Here's how the part is built. I have some questions about the finished solid (model axes, mm). A direction names the side the tool comes from. Coordinates: 2 decimals unless noted, no trailing zeros. Write each loop counter-clockwise with the first axis right and the second up, starting at its lowest first coordinate (ties: lowest second). Pieces come first, ordered by that corner, then holes.
```python
from build123d import *

# Parameters (mm, degrees)
F1_DEPTH = 136.652


with BuildPart() as f1:
    # F0 (on Front) → F1 (new body)
    with BuildSketch(Plane.XZ):
        with BuildLine():
            ThreePointArc((54.527499783, 20.9989734618), (54.7276679048, 20.7850152309), (54.9257769328, 20.5691490349))
            ThreePointArc((54.9257769328, 20.5691490349), (76.1901987299, 13.7983190429), (93.7294736505, 0))
            ThreePointArc((93.7294736505, 0), (99.5048519531, 7.4078439529), (104.1196596047, 15.589206731))
            ThreePointArc((104.1196596047, 15.589206731), (77.9936820742, 70.717129744), (25.6797344721, 102.1003335947))
            ThreePointArc((25.6797344721, 102.1003335947), (11.7801687474, 95.1325271586), (0, 84.9848240614))
            ThreePointArc((0, 84.9848240614), (8.2911620822, 73.9876177792), (13.9425107784, 61.4279930793))
            ThreePointArc((13.9425107784, 61.4279930793), (18.3589234819, 58.8669445911), (22.3165845225, 55.6419500772))
            ThreePointArc((22.3165845225, 55.6419500772), (45.1535066394, 46.1825872135), (54.6128695031, 23.3456650966))
            ThreePointArc((54.6128695031, 23.3456650966), (54.5915200165, 22.1715431248), (54.527499783, 20.9989734618))
        make_face()
        with BuildLine():
            ThreePointArc((93.7294736505, 0), (76.7382859544, -13.2702968374), (56.2774381887, -20.0640400021))
            ThreePointArc((56.2774381887, -20.0640400021), (56.3045635593, -20.8278500085), (56.3136070377, -21.5920880129))
            ThreePointArc((56.3136070377, -21.5920880129), (47.4391029946, -43.8287739455), (25.6927352215, -53.8448865624))
            ThreePointArc((25.6927352215, -53.8448865624), (19.5331456536, -59.5527538305), (12.1485373896, -63.5512351899))
            ThreePointArc((12.1485373896, -63.5512351899), (6.9976805403, -73.8751515766), (0, -83.0483213067))
            ThreePointArc((0, -83.0483213067), (12.9593131443, -94.1642757812), (28.4396211824, -101.3662410752))
            ThreePointArc((28.4396211824, -101.3662410752), (78.7986877851, -69.8190066246), (104.0530293111, -16.027912337))
            ThreePointArc((104.0530293111, -16.027912337), (99.5048519531, -7.6187369724), (93.7294736505, 0))
        make_face()
        with BuildLine():
            ThreePointArc((104.1196596047, 15.589206731), (99.5048519531, 7.4078439529), (93.7294736505, 0))
            ThreePointArc((93.7294736505, 0), (99.5048519531, -7.6187369724), (104.0530293111, -16.027912337))
            ThreePointArc((104.0530293111, -16.027912337), (104.9729816843, -8.0374124574), (105.2802302558, 0))
            ThreePointArc((105.2802302558, 0), (104.9896866841, 7.816173788), (104.1196596047, 15.589206731))
        make_face()
        with BuildLine():
            ThreePointArc((109.4791079844, -41.5241606534), (108.1075668029, -28.4905405885), (104.0530293111, -16.027912337))
            ThreePointArc((104.0530293111, -16.027912337), (78.7986877851, -69.8190066246), (28.4396211824, -101.3662410752))
            ThreePointArc((28.4396211824, -101.3662410752), (84.0593765341, -91.8939755487), (109.4791079844, -41.5241606534))
        make_face()
        with BuildLine():
            ThreePointArc((25.6797344721, 102.1003335947), (77.9936820742, 70.717129744), (104.1196596047, 15.589206731))
            ThreePointArc((104.1196596047, 15.589206731), (108.6056945653, 28.7097136295), (110.1253773364, 42.4924120307))
            ThreePointArc((110.1253773364, 42.4924120307), (83.3457717598, 94.174543643), (25.6797344721, 102.1003335947))
        make_face()
        with BuildLine():
            ThreePointArc((-56.3136070377, -21.5920880129), (-57.9095553347, -19.6725800372), (-59.3524805988, -17.6355408825))
            ThreePointArc((-59.3524805988, -17.6355408825), (-75.8807124036, -11.0348961584), (-89.8443087935, 0))
            ThreePointArc((-89.8443087935, 0), (-97.5622695247, -10.3588890688), (-102.9329187465, -22.1074901568))
            ThreePointArc((-102.9329187465, -22.1074901568), (-77.3108882291, -71.4629515478), (-30.118879838, -100.8800275576))
            ThreePointArc((-30.118879838, -100.8800275576), (-13.7568828123, -94.1642757812), (0, -83.0483213067))
            ThreePointArc((0, -83.0483213067), (-6.7178829074, -73.9195667822), (-11.6800359007, -63.7293191111))
            ThreePointArc((-11.6800359007, -63.7293191111), (-19.3289034102, -59.6979704443), (-25.6927352215, -53.8448865624))
            ThreePointArc((-25.6927352215, -53.8448865624), (-47.4391029946, -43.8287739455), (-56.3136070377, -21.5920880129))
        make_face()
        with BuildLine():
            ThreePointArc((-30.118879838, -100.8800275576), (-0.874115727, -105.2766014098), (28.4396211824, -101.3662410752))
            ThreePointArc((28.4396211824, -101.3662410752), (12.9593131443, -94.1642757812), (0, -83.0483213067))
            ThreePointArc((0, -83.0483213067), (-13.7568828123, -94.1642757812), (-30.118879838, -100.8800275576))
        make_face()
        with BuildLine():
            ThreePointArc((0, 84.9848240614), (11.7801687474, 95.1325271586), (25.6797344721, 102.1003335947))
            ThreePointArc((25.6797344721, 102.1003335947), (-0.7599031291, 105.2774877642), (-27.1509221895, 101.7189967851))
            ThreePointArc((-27.1509221895, 101.7189967851), (-12.4779975244, 95.1325271586), (0, 84.9848240614))
        make_face()
        with BuildLine():
            ThreePointArc((-102.9329187465, -22.1074901568), (-97.5622695247, -10.3588890688), (-89.8443087935, 0))
            ThreePointArc((-89.8443087935, 0), (-97.5622695247, 10.0482551584), (-103.0701310001, 21.4586807219))
            ThreePointArc((-103.0701310001, 21.4586807219), (-105.2797080994, -0.3315798868), (-102.9329187465, -22.1074901568))
        make_face()
        with BuildLine():
            ThreePointArc((-103.0701310001, 21.4586807219), (-97.5622695247, 10.0482551584), (-89.8443087935, 0))
            ThreePointArc((-89.8443087935, 0), (-75.8216360442, 11.2724103293), (-59.1261791661, 17.977953208))
            ThreePointArc((-59.1261791661, 17.977953208), (-57.0156534005, 20.7846782143), (-54.6128695031, 23.3456650966))
            ThreePointArc((-54.6128695031, 23.3456650966), (-45.1535066394, 46.1825872135), (-22.3165845225, 55.6419500772))
            ThreePointArc((-22.3165845225, 55.6419500772), (-18.1199759802, 59.0304671081), (-13.4179508285, 61.6732933224))
            ThreePointArc((-13.4179508285, 61.6732933224), (-7.9622593488, 74.0504399858), (0, 84.9848240614))
            ThreePointArc((0, 84.9848240614), (-12.4779975244, 95.1325271586), (-27.1509221895, 101.7189967851))
            ThreePointArc((-27.1509221895, 101.7189967851), (-76.4840523057, 72.3471950086), (-103.0701310001, 21.4586807219))
        make_face()
        with BuildLine():
            ThreePointArc((-102.9329187465, -22.1074901568), (-89.8443087935, -83.0483213067), (-30.118879838, -100.8800275576))
            ThreePointArc((-30.118879838, -100.8800275576), (-77.3108882291, -71.4629515478), (-102.9329187465, -22.1074901568))
        make_face()
        with BuildLine():
            ThreePointArc((-103.0701310001, 21.4586807219), (-76.4840523057, 72.3471950086), (-27.1509221895, 101.7189967851))
            ThreePointArc((-27.1509221895, 101.7189967851), (-89.8443087935, 84.9848240614), (-103.0701310001, 21.4586807219))
        make_face()
    extrude(amount=F1_DEPTH)


solid = f1.part
```
1) I need wall thicknesses on probe 1 along X at (y, z) = (-52.5, -45); probe 2 along Z at (x, y) = (-59, -54.5); probe 3 along X at (y, z) = (-68, -63). Which ranges of each line are inside material? Lowest first, please.
Values follow:
probe 1: x = -106 to -46.27, 46.27 to 109.38
probe 2: z = -101.06 to -18.16, 18.16 to 102.7
probe 3: x = -102.2 to -13.48, 13.48 to 105.68
2) On a 3-axis mill with a long thin cutter (end or side, diameter ignored), from which of +Z, -Z, +X, -X, +Y, -Y can I reach the whole of each face in a straight line? I mean faces 1 (the face through (-75.66, -67.37, -11.16)), 2 (the face through (48, -136.652, 49)). Say none if no direction works.
Values follow:
face 1: +Y, -Y
face 2: +Z, -Z, +X, -X, -Y
3) We'd pull the mould along Z, two halves only. Please class faces 3 (the face through (48, 0, 49)), 4 (the face through (-105.28, -67.37, -0.02)): pulls with the +Z half, pulls with the -Z half, needs draft (parallel to the pull), parting line crosses it, or undercut.
Values follow:
face 3: needs draft
face 4: undercut
4) Imagine slicing it at C-C on y = -43.5. Please give me the cut outline in (x, z), then the cut area to 3 significant figures.
Values follow:
outline: (-103.07, 21.46) arc R105.28 ccw to (-102.93, -22.11) arc R61.17 ccw to (-30.12, -100.88) arc R105.28 ccw to (28.44, -101.37) arc R62.61 ccw to (104.05, -16.03) arc R105.28 ccw to (104.12, 15.59) arc R63.26 ccw to (25.68, 102.1) arc R105.28 ccw to (-27.15, 101.72) arc R61.84 ccw to start; hole (-89.84, 0) arc R61.84 ccw to (-59.35, -17.64) arc R32.3 ccw to (-56.31, -21.59) arc R32.3 ccw to (-25.69, -53.84) arc R33.53 ccw to (-11.68, -63.73) arc R62.61 ccw to (0, -83.05) arc R61.17 ccw to (12.15, -63.55) arc R33.53 ccw to (25.69, -53.84) arc R32.3 ccw to (56.28, -20.06) arc R63.26 ccw to (93.73, 0) arc R62.61 ccw to (54.93, 20.57) arc R30.58 ccw to (54.53, 21) arc R32.3 ccw to (22.32, 55.64) arc R32.3 ccw to (13.94, 61.43) arc R61.84 ccw to (0, 84.98) arc R63.26 ccw to (-13.42, 61.67) arc R32.3 ccw to (-22.32, 55.64) arc R32.3 ccw to (-54.61, 23.35) arc R32.3 ccw to (-59.13, 17.98) arc R61.17 ccw to start
area: 27,000 mm2
5) Imagine slicing it at D-D on z = -89.5. Please give me the cut outline in (x, y).
Values follow:
outline: (-82.88, -136.65) - (87.1, -136.65) - (87.1, 0) - (-82.88, 0) - close
6) Imagine slicing it at B-B on z = -26.5. Please give me the cut outline in (x, y).
Values follow:
outline: (-104.22, -136.65) - (-55.94, -136.65) - (-55.94, 0) - (-104.22, 0) - close; (55.94, -136.65) - (107.65, -136.65) - (107.65, 0) - (55.94, 0) - close
7) Imagine slicing it at A-A on x = 60.5. Please give me the cut outline in (y, z), then the cut area to 3 significant figures.
Values follow:
outline: (-136.65, -102.64) - (0, -102.64) - (0, -19.28) - (-136.65, -19.28) - close; (-136.65, 19.59) - (0, 19.59) - (0, 104.27) - (-136.65, 104.27) - close
area: 23,000 mm2
8) Will these pins go through, and if not, where does the flat tip stop? pin 1 (10 mm diameter, centred on x = -63, y = -94, fed in from -Z); pin 2 (2 mm diameter, centred on y = -80.5, z = 71, fed in from +X); pin 3 (3 mm diameter, centred on x = -54.5, y = -71.5, fed in from -Z).
Values follow:
pin 1: stops at z = -101.28
pin 2: stops at x = 103.83
pin 3: stops at z = -102.16
